```python
from build123d import *

# Parameters (mm, degrees)
BOSS_EXTRUDE1_DEPTH = 9.525
SKETCH3_W           = 38.1
SKETCH3_H           = 20
BOSS_EXTRUDE2_DEPTH = 6.35


with BuildPart() as part:
    # Sketch2 → Boss-Extrude1 (new body, symmetric)
    with BuildSketch(Plane.XY):
        Polygon((-109.728, 0), (0, 0), (6.35, 0), (6.35, 32.766), (0, 32.766), (0, 6.35), (-109.728, 6.35), align=None)
    extrude(amount=BOSS_EXTRUDE1_DEPTH, both=True)

    # Sketch3 → Boss-Extrude2 (add)
    with BuildSketch(Plane.ZY):
        with Locations((0, 22.766)):
            Rectangle(SKETCH3_W, SKETCH3_H)
    extrude(amount=-BOSS_EXTRUDE2_DEPTH)


solid = part.part
```
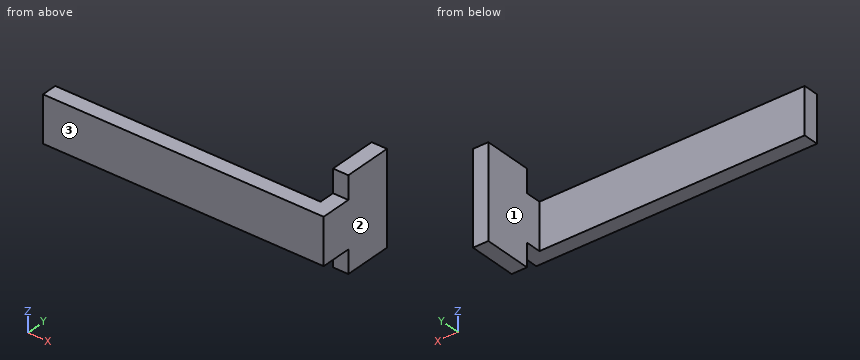
Source: CAD feature listing. Evaluate the final solid. Frame: model axes, mm. Face numbers are marked on the shaded views. Give positions to 0.01 mm unless a question says otherwise; leave off trailing zeros. Loops run counter-clockwise (first coordinate to the right, second up) from the corner with the lowest first, then second, coordinate; pieces in that order, holes last. Notation, with made-up numbers: (89, 11) -> (106, 11) arc R33 cw to (106, 49) -> close; hole circle Ø7 at (62.25, -12.5). An arc over 180 degrees is marked (long way). Use a Markdown table: item, result. Add a question column.
(1) Section query B-B (z = 8). Output: boundary loops of the cut face in (x, y), then the cut area to 3 significant figures.
(2) Ray query, line 1 (Y direction, x = -52, z = -8); line 2 (Z direction, x = -80, y = 2.5) (3 decimals). Return the intervals inside material, ascending.
(3) Pull-direction query (X, two-part tool) for the marked faces 1, 2 and 3; classes: +X half, -X half, draft (parallel to the pull), parting line (faces both ways), or undercut.
(4) Section query A-A (y = 4). Output: boundary loops of the cut face in (x, z) (3 decimals), then the cut area to 3 significant figures.
(5) First-contact query: pin 1 Ø3 at (x, z) = (3, -15.5) entering from -Y; pin 2 Ø5.5 at (x, z) = (-81.5, -0.5) entering from +Y; pin 3 Ø4 at (x, y) = (-27.5, 5) entering from -Z (3 decimals). Flat tips, straight axial feed; report the tip coordinate or a pass-through.
(6) Section query C-C (x = -3). Output: boundary loops of the cut face in (y, z) (3 decimals).
Checked values:
| question | item | result |
|---|---|---|
| 1 | outline | (-109.73, 0) -> (6.35, 0) -> (6.35, 32.77) -> (0, 32.77) -> (0, 6.35) -> (-109.73, 6.35) -> close |
| 1 | area | 905 mm^2 |
| 2 | line 1 | 0 to 6.35 |
| 2 | line 2 | -9.525 to 9.525 |
| 3 | face 1 | -X half |
| 3 | face 2 | +X half |
| 3 | face 3 | draft |
| 4 | outline | (-109.728, -9.525) -> (6.35, -9.525) -> (6.35, 9.525) -> (-109.728, 9.525) -> close |
| 4 | area | 2,210 mm^2 |
| 5 | pin 1 | y = 12.77 |
| 5 | pin 2 | y = 6.35 |
| 5 | pin 3 | z = -9.525 |
| 6 | outline | (0, -9.525) -> (6.35, -9.525) -> (6.35, 9.525) -> (0, 9.525) -> close |
